Read the model definition and answer for the solid it produces. Units are mm, in the model's axes. Face numbers are marked on the shaded views. A direction names the side the tool comes from. Coordinates: 2 decimals unless noted, no trailing zeros. Loops run counter-clockwise (first coordinate to the right, second up) from the corner with the lowest first, then second, coordinate; pieces in that order, holes last. Notation, with made-up numbers: (89.5, -2.75) -> (107.5, -2.75) arc R10 cw to (107.5, 1.25) -> close; hole circle Ø10 at (32, -37). An arc over 180 degrees is marked (long way). Answer as a JSON object with one key per item and string values. Group by question number.
1) Which of the six approach directions +Z, -Z, +X, -X, +Y, -Y give full straight-line access (tool end or side, diameter ignored) to the marked faces 1, 2 and 3?
2) Flat-ended cylindrical pins translate along their axes: P1, Ø4, axis at x = 1, y = 5.5, coming from the -Z side; P2, Ø3, axis at x = 15.5, y = 15.5, coming from the -Z side; P3, Ø3, axis at y = -3.5, z = 10.5, coming from the +X side; P4, Ø4, axis at y = -6, z = 2.5, coming from the -X side. Find the tip coordinate at first contact, or state that the pin passes through.
3) Consider probe 1 along Y at (x, z) = (0, 6); probe 2 along X at (y, z) = (-0.5, 5.75); probe 3 along X at (y, z) = (-3, 12.5). Determine where each line is inside the solid, lowest interval first. Write a range as [from, to].
4) Section A-A, the plane y = 0 is taken. Give the vertices of the cut face in (x, z), plus the area to 3 significant figures.
5) Section D-D, the plane x = 16 is taken. Give the vertices of the cut face in (y, z).
6) Section B-B, the plane z = 3.5 is taken. Give the vertices of the cut face in (x, y).
7) Determine the mould class of the marked faces 4, 5 and 6 for opening direction X: released by +X, released by -X, zero draft, split by the parting line, or undercut.
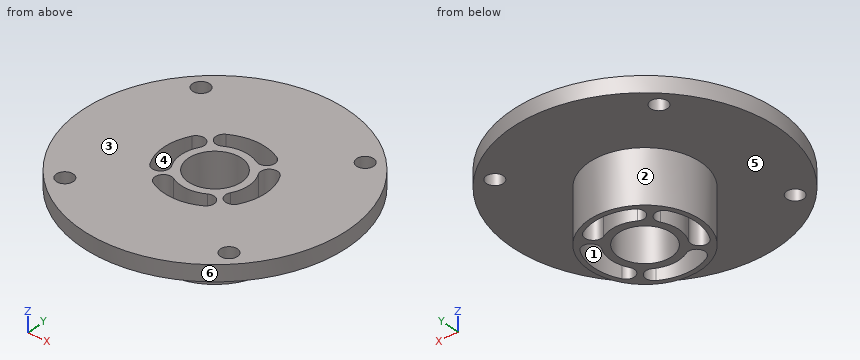
from build123d import *

# Parameters (mm, degrees)
SKETCH_R        = 10.5
PAD_DEPTH       = 10
SKETCH001_R     = 25
SKETCH001_R_2   = 1.6
PAD001_DEPTH    = 3
SKETCH002_R     = 5
POCKET_DEPTH    = 13.001
POCKET001_DEPTH = 13.001


with BuildPart() as part:
    # Sketch → Pad (new body)
    with BuildSketch(Plane.XY):
        Circle(SKETCH_R)
    extrude(amount=PAD_DEPTH)

    # Sketch001 (on Face3 of Pad) → Pad001 (join)
    with BuildSketch(Plane.XY.offset(10)):
        Circle(SKETCH001_R)
        with Locations((-15.5, -15.5)):
            Circle(SKETCH001_R_2, mode=Mode.SUBTRACT)
        with Locations((15.5, -15.5)):
            Circle(SKETCH001_R_2, mode=Mode.SUBTRACT)
        with Locations((15.5, 15.5)):
            Circle(SKETCH001_R_2, mode=Mode.SUBTRACT)
        with Locations((-15.5, 15.5)):
            Circle(SKETCH001_R_2, mode=Mode.SUBTRACT)
    extrude(amount=PAD001_DEPTH)

    # Sketch002 (on Face3 of Pad001) → Pocket (cut, through all)
    with BuildSketch(Plane.XY.offset(13)):
        Circle(SKETCH002_R)
    extrude(amount=-POCKET_DEPTH, mode=Mode.SUBTRACT)

    # Sketch003 (on Face3 of Pocket) → Pocket001 (cut, through all)
    with BuildSketch(Plane.XY.offset(13)):
        with BuildLine():
            ThreePointArc((3.2, 5.542563), (5.385641, 6.128203), (4.8, 8.313844))
            ThreePointArc((4.8, 8.313844), (0, 9.6), (-4.8, 8.313844))
            ThreePointArc((-4.8, 8.313844), (-5.385641, 6.128203), (-3.2, 5.542563))
            ThreePointArc((3.2, 5.542563), (0, 6.4), (-3.2, 5.542563))
        make_face()
        with BuildLine():
            ThreePointArc((8.313844, 4.8), (6.128203, 5.385641), (5.542563, 3.2))
            ThreePointArc((5.542563, -3.2), (6.4, 0), (5.542563, 3.2))
            ThreePointArc((5.542563, -3.2), (6.128203, -5.385641), (8.313844, -4.8))
            ThreePointArc((8.313844, -4.8), (9.6, 0), (8.313844, 4.8))
        make_face()
        with BuildLine():
            ThreePointArc((-5.542563, 3.2), (-6.128203, 5.385641), (-8.313844, 4.799999))
            ThreePointArc((-8.313844, 4.799999), (-9.6, 0), (-8.313844, -4.799999))
            ThreePointArc((-8.313844, -4.799999), (-6.128203, -5.385641), (-5.542563, -3.199999))
            ThreePointArc((-5.542563, 3.2), (-6.4, 0), (-5.542563, -3.199999))
        make_face()
        with BuildLine():
            ThreePointArc((4.8, -8.313844), (5.385641, -6.128203), (3.2, -5.542563))
            ThreePointArc((-3.199999, -5.542563), (0, -6.4), (3.2, -5.542563))
            ThreePointArc((-3.199999, -5.542563), (-5.38564, -6.128203), (-4.8, -8.313844))
            ThreePointArc((-4.8, -8.313844), (0, -9.6), (4.8, -8.313844))
        make_face()
    extrude(amount=-POCKET001_DEPTH, mode=Mode.SUBTRACT)


solid = part.part
Determined:
{
 "1": {"face 1": "+Z, -Z", "face 2": "-Z", "face 3": "+Z, +X, -X, +Y, -Y"},
 "2": {"P1": "z = 0", "P2": "through", "P3": "x = 24.92", "P4": "x = -9.71"},
 "3": {"probe 1": "[-10.5, -9.6], [-6.4, -5], [5, 6.4], [9.6, 10.5]", "probe 2": "[-10.49, -9.59], [-6.38, -4.97], [4.97, 6.38], [9.59, 10.49]", "probe 3": "[-24.82, -9.12], [-5.65, -4], [4, 5.65], [9.12, 24.82]"},
 "4": {"outline": "(-25, 10) -> (-10.5, 10) -> (-10.5, 0) -> (-9.6, 0) -> (-9.6, 13) -> (-25, 13) -> close; (-6.4, 0) -> (-5, 0) -> (-5, 13) -> (-6.4, 13) -> close; (5, 0) -> (6.4, 0) -> (6.4, 13) -> (5, 13) -> close; (9.6, 0) -> (10.5, 0) -> (10.5, 10) -> (25, 10) -> (25, 13) -> (9.6, 13) -> close", "area": "147 mm²"},
 "5": {"outline": "(-19.21, 10) -> (-17.02, 10) -> (-17.02, 13) -> (-19.21, 13) -> close; (-13.98, 10) -> (13.98, 10) -> (13.98, 13) -> (-13.98, 13) -> close; (17.02, 10) -> (19.21, 10) -> (19.21, 13) -> (17.02, 13) -> close"},
 "6": {"outline": "circle Ø21 at (0, 0); hole (-8.31, -4.8) arc R1.6 ccw to (-5.54, -3.2) arc R6.4 cw to (-5.54, 3.2) arc R1.6 ccw to (-8.31, 4.8) arc R9.6 ccw to start; hole circle Ø10 at (0, 0); hole (-4.8, -8.31) arc R9.6 ccw to (4.8, -8.31) arc R1.6 ccw to (3.2, -5.54) arc R6.4 cw to (-3.2, -5.54) arc R1.6 ccw to start; hole (-4.8, 8.31) arc R1.6 ccw to (-3.2, 5.54) arc R6.4 cw to (3.2, 5.54) arc R1.6 ccw to (4.8, 8.31) arc R9.6 ccw to start; hole (5.54, -3.2) arc R1.6 ccw to (8.31, -4.8) arc R9.6 ccw to (8.31, 4.8) arc R1.6 ccw to (5.54, 3.2) arc R6.4 cw to start"},
 "7": {"face 4": "undercut", "face 5": "zero draft", "face 6": "split by the parting line"}
}
